Can you work these out from the model? Positions are in its coordinate system, mm. A direction names the side the tool comes from. Give positions to 0.01 mm unless a question says otherwise; leave off trailing zeros. Write each loop counter-clockwise with the first axis right and the second up, starting at its lowest first coordinate (ties: lowest second). Pieces come first, ordered by that corner, then holes. Notation, with made-up numbers: (14, 16) -> (69, 16) arc R31 ccw to (69, 48) -> close; hole circle Ø7 at (28, 13). An arc over 180 degrees is marked (long way). One line per item, written item: value.
from build123d import *

# Parameters (mm, degrees)
SKETCH1_W           = 78.232
SKETCH1_H           = 55.88
BOSS_EXTRUDE1_DEPTH = 5.6388
SKETCH2_W           = 78.232
SKETCH2_H           = 26.67
BOSS_EXTRUDE2_DEPTH = 38.1
BOSS_EXTRUDE2_TAPER = 8
CUT_EXTRUDE1_DEPTH  = 19.05


with BuildPart() as part:
    # Sketch1 → Boss-Extrude1 (new body)
    with BuildSketch(Plane(origin=(0, 0, 0), x_dir=(1, 0, 0), z_dir=(0, 1, 0))):
        Rectangle(SKETCH1_W, SKETCH1_H)
    extrude(amount=BOSS_EXTRUDE1_DEPTH)

    # Sketch2 → Boss-Extrude2 (add)
    with BuildSketch(Plane(origin=(0, 5.6388, 0), x_dir=(1, 0, 0), z_dir=(0, 1, 0))):
        Rectangle(SKETCH2_W, SKETCH2_H)
    extrude(amount=BOSS_EXTRUDE2_DEPTH, taper=BOSS_EXTRUDE2_TAPER)

    # 3DSketch1 → Cut-Extrude1 (cut, symmetric)
    with BuildSketch(Plane(origin=(39.116, 28.335306521, -1e-09), x_dir=(-0.9811621581078611, 0.1931859712741186, 2.0390368677299597e-12), z_dir=(2.078300433678865e-12, 0, 1.0))):
        Polygon((0, 0), (12.678292519, -8.831750582), (34.020347529, 21.805529518), (33.186170505, 26.042187717), (45.646929913, 28.495649552), (63.27719365, 10.210852573), (75.090838988, 23.581993737), (79.734016802, 0), (2.975738849, -15.113324905), align=None)
    extrude(amount=CUT_EXTRUDE1_DEPTH, both=True, mode=Mode.SUBTRACT)


solid = part.part
1) I need wall thicknesses on L1, parallel to Y at x = -15, z = 15.5; L2, parallel to X at y = 23, z = -4; L3, parallel to Y at x = -2, z = -2.5. Which ranges of each line are inside material? Lowest first, please.
Answer list:
L1: y = 0 to 5.64
L2: x = -34.81 to -20.08, 11.35 to 36.68
L3: y = 0 to 9.19
2) Will these pins go through, and if not, where does the flat tip stop? pin 1 (10 mm diameter, centred on x = -8.5, z = -20.5, fed in from -Y); pin 2 (12 mm diameter, centred on y = 29.5, z = -3, fed in from -X); pin 3 (4.5 mm diameter, centred on x = 9.5, z = -20, fed in from +Y); pin 4 (10 mm diameter, centred on y = 31, z = 7.5, fed in from +X).
Answer list:
pin 1: stops at y = 0
pin 2: stops at x = -34.15
pin 3: stops at y = 5.64
pin 4: stops at x = 36.25
3) We'd pull the mould along X, two halves only. Please class faces 4 (the face through (-39.116, 3, 0)), 5 (the face through (31.932, 35.775, 0.134)), 6 (the face through (15.14, 26.66, 0.17)): released by +X, released by -X, zero draft, split by the parting line, or undercut.
Answer list:
face 4: released by -X
face 5: released by +X
face 6: undercut
4) If we section it at A-A (z = -22.5): Write out the boundary of the cut face in (x, y), and give its area (3 significant figures).
Answer list:
outline: (-39.12, 0) -> (39.12, 0) -> (39.12, 5.64) -> (-39.12, 5.64) -> close
area: 441 mm^2
5) For faces 1 (the face through (-1, 5.639, -21)), 2 (the face through (-1, 5.639, 21)), 3 (the face through (1.524, 11, 0)), which set-ups out of +Z, -Z, +X, -X, +Y, -Y let a thin tool reach every point of the face, with its end or its side?
Answer list:
face 1: -Z, +X, -X, +Y
face 2: +Z, +X, -X, +Y
face 3: +Z, -Z, +Y
